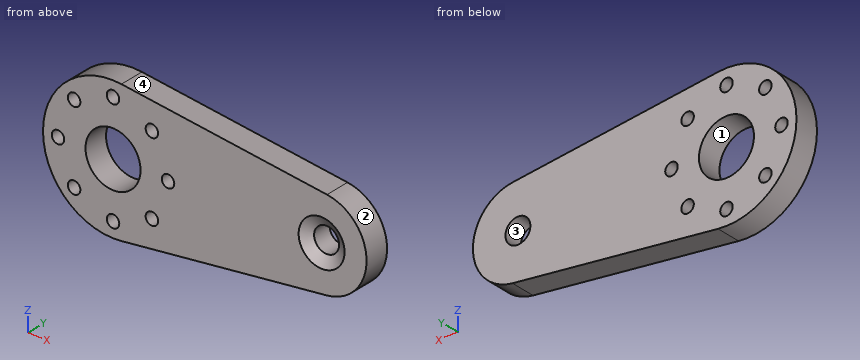
```python
from build123d import *

# Parameters (mm, degrees)
F0_R     = 1.25
F0_R_2   = 5.5
F0_R_3   = 2.5
F1_DEPTH = 5
F2_SIZE2 = 2.09
F2_SIZE  = 1.223


with BuildPart() as f1:
    # F0 (on Front) → F1 (new body)
    with BuildSketch(Plane.XZ):
        with BuildLine():
            Line((20.093722, 8.935112), (-21.020701, 13.899064))
            ThreePointArc((-21.020701, 13.899064), (-36.698805, 0), (-21.020701, -13.899064))
            Line((-21.020701, -13.899064), (20.093722, -8.935112))
            ThreePointArc((20.093722, -8.935112), (28.014941, 0), (20.093722, 8.935112))
        make_face()
        with Locations((-22.698805, -11)):
            Circle(F0_R, mode=Mode.SUBTRACT)
        with Locations((-30.47698, -7.778175)):
            Circle(F0_R, mode=Mode.SUBTRACT)
        with Locations((-14.92063, -7.778175)):
            Circle(F0_R, mode=Mode.SUBTRACT)
        with Locations((-33.698805, 0)):
            Circle(F0_R, mode=Mode.SUBTRACT)
        with Locations((-22.698805, 0)):
            Circle(F0_R_2, mode=Mode.SUBTRACT)
        with Locations((-11.698805, 0)):
            Circle(F0_R, mode=Mode.SUBTRACT)
        with Locations((-30.47698, 7.778175)):
            Circle(F0_R, mode=Mode.SUBTRACT)
        with Locations((-22.698805, 11)):
            Circle(F0_R, mode=Mode.SUBTRACT)
        with Locations((-14.92063, 7.778175)):
            Circle(F0_R, mode=Mode.SUBTRACT)
        with Locations((19.014941, 0)):
            Circle(F0_R_3, mode=Mode.SUBTRACT)
    extrude(amount=F1_DEPTH)

    # F2
    f2_edges = [f1.edges().sort_by_distance(p)[0] for p in [
        (16.514941, -5, 0),
    ]]
    chamfer(f2_edges, length=F2_SIZE, length2=F2_SIZE2)


solid = f1.part
```
Check sheet for the modelled part. Datum: model origin and axes. Units: mm. Face numbers are marked on the shaded views. Coordinates: 2 decimals unless noted, no trailing zeros. Order: outer loops, then holes, each group sorted by start corner. A loop starts at its lowest first (then second) coordinate and runs counter-clockwise, first axis right, second up. Notation, with made-up numbers: (33.25, 33) -> (83.25, 33) arc R28 cw to (83.25, 68) -> close; hole circle Ø4 at (5, 70.25). An arc over 180 degrees is marked (long way). Write item = value, one per line. Start each with the question number.
1) Material ranges on L1, parallel to X at y = -0.35, z = 0.5; L2, parallel to Z at x = -14, y = -0.9; L3, parallel to X at y = -4.45, z = 2.5, recorded low to high.
2) Go/stop test with flat-tipped pins: P1, Ø2, axis at y = -1.5, z = 3.5, coming from the -X side; P2, Ø1.5, axis at y = -3, z = 9, coming from the -X side; P3, Ø3, axis at y = -2, z = -10, coming from the -X side. Record where each tip stops, or that it passes through.
3) Cross-section at B-B (z = 11). Enter the section's corners in (x, y).
4) Cross-section at C-C (y = -1.45). State how many separate pieces and enclosed holes the cut face has, then the cut area to 3 significant figures.
5) Cross-section at A-A (x = -26.5). Enter the section's corners in (y, z).
6) Mould release check, pull along Z, two halves, no side actions. Record for the marked faces 1, 2, 3 and 4: +Z half, -Z half, draft (parallel to the pull), parting line (faces both ways), or undercut.
Ans:
q1.L1 = -36.69 to -34.84, -32.55 to -28.18, -17.22 to -12.84, -10.55 to 16.57, 21.46 to 28
q1.L2 = -13.05 to -8.62, -6.93 to 6.93, 8.62 to 13.05
q1.L3 = -36.47 to -27.6, -17.8 to 16.36, 21.67 to 27.66
q2.P1 = -36.47
q2.P2 = -34.01
q2.P3 = -33.82
q3.outline = (-31.36, -5) -> (-23.95, -5) -> (-23.95, 0) -> (-31.36, 0) -> close; (-21.45, -5) -> (2.99, -5) -> (2.99, 0) -> (-21.45, 0) -> close
q4.separate_pieces = 1
q4.enclosed_holes = 10
q4.area = 1,250 mm²
q5.outline = (-5, -13.47) -> (0, -13.47) -> (0, -3.98) -> (-5, -3.98) -> close; (-5, 3.98) -> (0, 3.98) -> (0, 13.47) -> (-5, 13.47) -> close
q6.face_1 = undercut
q6.face_2 = parting line
q6.face_3 = undercut
q6.face_4 = +Z half
